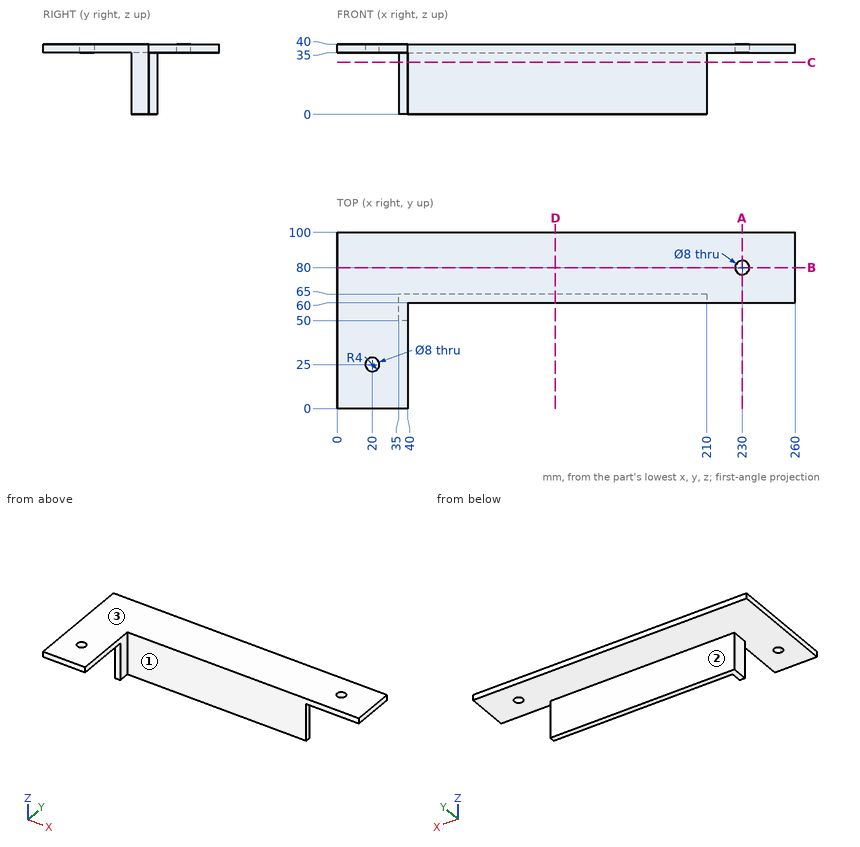
Answer from the drawing. Dimensions are ordinates in mm from the lowest x, y and z of the part. A direction names the side the tool comes from. Coordinates: 2 decimals unless noted, no trailing zeros. Order: outer loops, then holes, each group sorted by start corner. A loop starts at its lowest first (then second) coordinate and runs counter-clockwise, first axis right, second up. Notation, with made-up numbers: (59, 45.5) - (94, 45.5) arc R22 ccw to (94, 64.5) - close; hole circle Ø1 at (15, 63.25). An arc over 180 degrees is marked (long way). Put each result on its own line as item: value. Start each with the question number.
1) Flat-ended cylindrical pins translate along their axes: pin 1 (8 mm diameter, centred on x = 207, y = 75.5, fed in from -Z); pin 2 (2 mm diameter, centred on x = 175, z = 18, fed in from -Y); pin 3 (2 mm diameter, centred on x = 181.5, z = 14.5, fed in from +Y); pin 4 (20 mm diameter, centred on y = 39.5, z = 24, fed in from +X). Find the tip coordinate at first contact, or state that the pin passes through.
2) Find section C-C (z = 29.5). Give the vertices of the cut face in (x, y), plus the area to 3 significant figures.
3) Find the intervals of material crossed by line 1 (Y direction, x = 20, z = 38.75); line 2 (Y direction, x = 230, z = 38); line 3 (X direction, y = 25, z = 36), in increasing order. Write a range as from..to.
4) For the marked faces 1, 2 and 3, determine the directions among +Z, -Z, +X, -X, +Y, -Y from which every point of the face is accessible in a straight line to the end or side of a thin tool.
5) Find section D-D (x = 124). Give the vertices of the cut face in (y, z), plus the area to 3 significant figures.
6) Find section B-B (y = 80). Give the vertices of the cut face in (x, z).
7) Find section A-A (x = 230). Give the vertices of the cut face in (y, z), plus the area to 3 significant figures.
Results list:
1. pin 1: stops at z = 35
1. pin 2: stops at y = 60
1. pin 3: stops at y = 65
1. pin 4: passes through
2. outline: (35, 50) - (40, 50) - (40, 60) - (210, 60) - (210, 65) - (35, 65) - close
2. area: 925 mm^2
3. line 1: y = 0..21, 29..100
3. line 2: y = 60..76, 84..100
3. line 3: x = 0..16, 24..40
4. face 1: +Z, -Z, +X, -Y
4. face 2: -Z, +X, -X, +Y
4. face 3: +Z, +X, -X, +Y, -Y
5. outline: (60, 0) - (65, 0) - (65, 35) - (100, 35) - (100, 40) - (60, 40) - close
5. area: 375 mm^2
6. outline: (0, 35) - (226, 35) - (226, 40) - (0, 40) - close; (234, 35) - (260, 35) - (260, 40) - (234, 40) - close
7. outline: (60, 35) - (76, 35) - (76, 40) - (60, 40) - close; (84, 35) - (100, 35) - (100, 40) - (84, 40) - close
7. area: 160 mm^2
